Part print with two shaded views. Sizes in mm from the minimum x, y, z corner. Round coordinates to 2 decimals unless told otherwise and drop trailing zeros. Loops run counter-clockwise (first coordinate to the right, second up) from the corner with the lowest first, then second, coordinate; pieces in that order, holes last. Notation, with made-up numbers: (69.5, 86.25) - (96.5, 86.25) arc R28 ccw to (96.5, 108.25) - close; hole circle Ø2 at (49, -39.75). An arc over 180 degrees is marked (long way). Use a Markdown table: item, result.
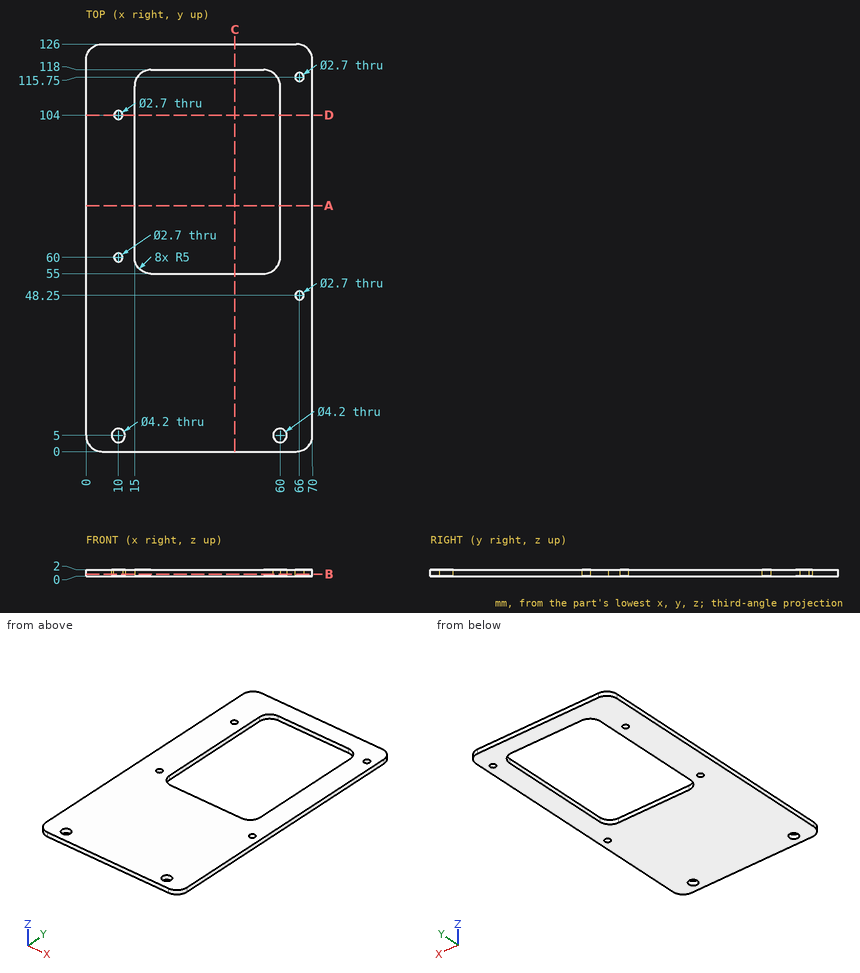
Q1. Cut at B-B, the plane z = 0.6. List the corners of the cut face in (x, y).
Results found:
| item | result |
|---|---|
| outline | (0, 5) arc R5 ccw to (5, 0) - (65, 0) arc R5 ccw to (70, 5) - (70, 121) arc R5 ccw to (65, 126) - (5, 126) arc R5 ccw to (0, 121) - close; hole circle Ø4.2 at (10, 5); hole circle Ø2.7 at (10, 60); hole circle Ø2.7 at (10, 104); hole (15, 60) arc R5 ccw to (20, 55) - (55, 55) arc R5 ccw to (60, 60) - (60, 113) arc R5 ccw to (55, 118) - (20, 118) arc R5 ccw to (15, 113) - close; hole circle Ø4.2 at (60, 5); hole circle Ø2.7 at (66, 48.25); hole circle Ø2.7 at (66, 115.75) |
Q2. Cut at A-A, the plane y = 76. List the corners of the cut face in (x, z), plus the area to 3 significant figures.
Results found:
| item | result |
|---|---|
| outline | (0, 0) - (15, 0) - (15, 2) - (0, 2) - close; (60, 0) - (70, 0) - (70, 2) - (60, 2) - close |
| area | 50.0 mm2 |
Q3. Cut at C-C, the plane x = 46. List the corners of the cut face in (y, z).
Results found:
| item | result |
|---|---|
| outline | (0, 0) - (55, 0) - (55, 2) - (0, 2) - close; (118, 0) - (126, 0) - (126, 2) - (118, 2) - close |
Q4. Probe line 1 (Y direction, x = 10, z = 0.95); line 2 (X direction, y = 104, z = 1.5); line 3 (Y direction, x = 26.5, z = 1.95). List the from-to ranges inside material, lowest first.
Results found:
| item | result |
|---|---|
| line 1 | y = 0 to 2.9, 7.1 to 58.65, 61.35 to 102.65, 105.35 to 126 |
| line 2 | x = 0 to 8.65, 11.35 to 15, 60 to 70 |
| line 3 | y = 0 to 55, 118 to 126 |
Q5. Cut at D-D, the plane y = 104. List the corners of the cut face in (x, z).
Results found:
| item | result |
|---|---|
| outline | (0, 0) - (8.65, 0) - (8.65, 2) - (0, 2) - close; (11.35, 0) - (15, 0) - (15, 2) - (11.35, 2) - close; (60, 0) - (70, 0) - (70, 2) - (60, 2) - close |
Q6. Drop a flat-ended pin along its axis: pin 1 (0.6 mm diameter, centred on y = 90.5, z = 1, fed in from -X). Give the stop position or say it passes through.
Results found:
| item | result |
|---|---|
| pin 1 | stops at x = 0 |
